The listing builds one solid part. Answer for the finished solid, in the listing's coordinates (mm). Round coordinates to 2 decimals unless told otherwise and drop trailing zeros. Write each loop counter-clockwise with the first axis right and the second up, starting at its lowest first coordinate (ties: lowest second). Pieces come first, ordered by that corner, then holes. Notation, with made-up numbers: M -19,13.25 L -10,13.25 A29 ccw -10,45.25 Z; hole C -35,-24.75 d9. An arc over 180 degrees is marked long. Put each result on its own line as item: value. Start each with the question number.
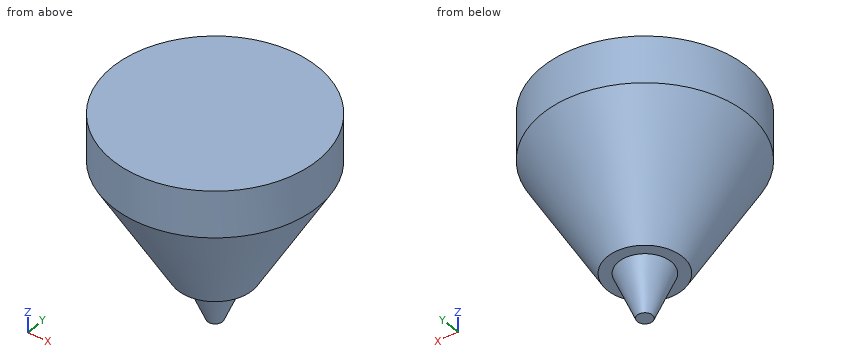
```python
from build123d import *

# Parameters (mm, degrees)
ESQUISSE2_R             = 15.4
ENL_V_MAT_EXTRU_1_DEPTH = 54


with BuildPart() as part:
    # Esquisse1 → Révolution1 (revolve)
    with BuildSketch(Plane(origin=(0, 0, 0), x_dir=(0, 0, -1), z_dir=(1, 0, 0))):
        Polygon((-30.55, 10.985938257), (-35.55, 10.985938257), (-35.55, 0), (35.55, 0), (35.55, 15.4), (30.55, 15.4), (-18.45, 4), align=None)
    revolve(axis=Axis((0, 0, 35.55), (0, 0, -1)))

    # Esquisse2 → Enlèv. mat.-Extru.1 (cut)
    with BuildSketch(Plane.XY.offset(18.45)):
        Circle(ESQUISSE2_R)
    extrude(amount=-ENL_V_MAT_EXTRU_1_DEPTH, mode=Mode.SUBTRACT)

    # Esquisse6 → Révolution2 (revolve)
    with BuildSketch(Plane(origin=(0, 0, 0), x_dir=(0, 0, -1), z_dir=(1, 0, 0))):
        Polygon((-18.45, 2.8), (-13.65, 0.8), (-13.65, 0), (-18.45, 0), align=None)
    revolve(axis=Axis((0, 0, 13.65), (0, 0, 1)))


solid = part.part
```
Item 1: Flat-ended cylindrical pins translate along their axes: pin 1 (3 mm diameter, centred on x = 4.5, z = 26.5, fed in from -Y); pin 2 (6 mm diameter, centred on x = 3, y = -3.5, fed in from -Z); pin 3 (1 mm diameter, centred on y = -4, z = 26.5, fed in from +X). Find the tip coordinate at first contact, or state that the pin passes through.
Item 2: Section A-A (y = 0) is taken. Give the vertices of the cut face in (x, z).
Item 3: Section C-C (z = 32.25) is taken. Give the vertices of the cut face in (x, y), and give its area (3 significant figures).
Item 4: Consider line 1 along X through (y, z) = (-0.25, 34); line 2 along Z through (x, y) = (2, -8); line 3 along Z through (x, y) = (-7.25, -2.5). Determine where each line is inside the solid, lowest interval first. Write a range as [from, to].
Item 5: Section D-D (z = 17.5) is taken. Give the vertices of the cut face in (x, y), and give its area (3 significant figures).
Output values:
1. pin 1: stops at y = -8.62
1. pin 2: stops at z = 15.59
1. pin 3: stops at x = 8.07
2. outline: M -10.99,30.55 L -4,18.45 L -2.8,18.45 L -0.8,13.65 L 0.8,13.65 L 2.8,18.45 L 4,18.45 L 10.99,30.55 L 10.99,35.55 L -10.99,35.55 Z
3. outline: C 0,0 d21.97
3. area: 379 mm^2
4. line 1: x = [-10.98, 10.98]
4. line 2: z = [25.8, 35.55]
4. line 3: z = [24.8, 35.55]
5. outline: C 0,0 d4.81
5. area: 18.2 mm^2
